from build123d import *

# Parameters (mm, degrees)
EXTRUDE_1_DEPTH     = 4
FILLET_1_R          = 0.5
FILLET_2_R          = 1
CUT_EXTRUDE_1_DEPTH = 0.5
SKETCH_3_W          = 3.444181234
SKETCH_3_H          = 7
SKETCH_3_W_2        = 2.596632025
CUT_EXTRUDE_2_DEPTH = 17


with BuildPart() as part:
    # 草图1 → 凸台-拉伸1 (new, symmetric)
    with BuildSketch(Plane.XY):
        Polygon((0, 0), (6.275985866, 3.1), (14.2, 2), (14.2, 20), (14.7, 20), (14.7, 1.425796077), (6.359548127, 2.583605352), (1.1290092, 0), (6.359548127, -2.583605352), (14.7, -1.425796077), (14.7, -20), (14.2, -20), (14.2, -2), (6.275985866, -3.1), align=None)
    extrude(amount=EXTRUDE_1_DEPTH, both=True)

    # 圆角1
    fillet_1_edges = [part.edges().sort_by_distance(p)[0] for p in [
        (14.2, 2, 0),
        (6.359548127, 2.583605352, 0),
        (1.1290092, 0, 0),
        (6.359548127, -2.583605352, 0),
        (14.2, -2, 0),
    ]]
    fillet(fillet_1_edges, radius=FILLET_1_R)

    # 圆角2
    fillet_2_edges = [part.edges().sort_by_distance(p)[0] for p in [
        (0, 0, 0),
        (6.275985866, 3.1, 0),
        (14.7, 1.425796077, 0),
        (14.7, -1.425796077, 0),
        (6.275985866, -3.1, 0),
    ]]
    fillet(fillet_2_edges, radius=FILLET_2_R)

    # 草图2 → 切除-拉伸1 (cut)
    with BuildSketch(Plane.ZY.offset(-14.2)):
        with BuildLine():
            Line((1.5, 16), (1.5, 12))
            ThreePointArc((1.5, 12), (0, 10.5), (-1.5, 12))
            Line((-1.5, 12), (-1.5, 16))
            ThreePointArc((-1.5, 16), (0, 17.5), (1.5, 16))
        make_face()
        with BuildLine():
            Line((1.5, -12), (1.5, -16))
            ThreePointArc((1.5, -16), (0, -17.5), (-1.5, -16))
            Line((-1.5, -16), (-1.5, -12))
            ThreePointArc((-1.5, -12), (0, -10.5), (1.5, -12))
        make_face()
    extrude(amount=-CUT_EXTRUDE_1_DEPTH, mode=Mode.SUBTRACT)

    # 草图3 → 切除-拉伸2 (cut, symmetric)
    with BuildSketch(Plane.ZY.offset(-14.2)):
        with Locations((4.722090617, 0)):
            Rectangle(SKETCH_3_W, SKETCH_3_H)
        with Locations((-4.298316013, 0)):
            Rectangle(SKETCH_3_W_2, SKETCH_3_H)
    extrude(amount=CUT_EXTRUDE_2_DEPTH, both=True, mode=Mode.SUBTRACT)


solid = part.part
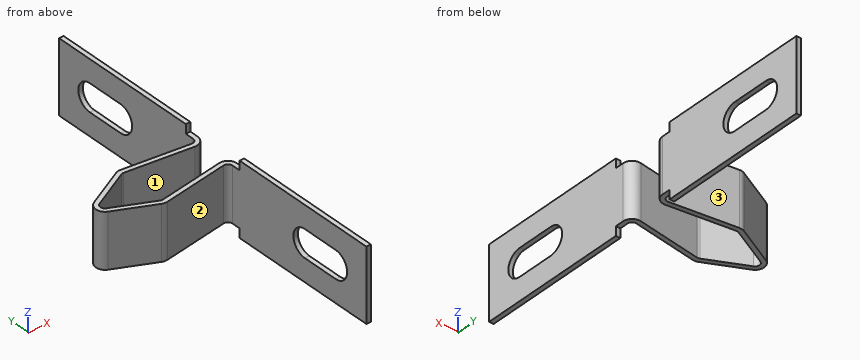
The listing builds one solid part. Answer for the finished solid, in the listing's coordinates (mm). Face numbers are marked on the shaded views. A direction names the side the tool comes from. Round coordinates to 2 decimals unless told otherwise and drop trailing zeros. Loops run counter-clockwise (first coordinate to the right, second up) from the corner with the lowest first, then second, coordinate; pieces in that order, holes last. Notation, with made-up numbers: M 56,-33.5 L 86,-33.5 A15 cw 86,-7.5 Z; hole C 18,-14 d8. An arc over 180 degrees is marked long. Return JSON: item names as keys, results as strings.
Q1. Find section B-B, the plane y = -17. Determine the outline of the cut face in (x, z), plus the area to 3 significant figures.
Results list:
{"outline": "M 14.2,-4 L 14.7,-4 L 14.7,-1.12 L 14.2,-1.12 Z; M 14.2,1.12 L 14.7,1.12 L 14.7,4 L 14.2,4 Z", "area": "2.88 mm2"}
Q2. Each of these flat-tipped pins is pushed along its axis until it touches: pin 1 Ø2 at (x, y) = (8.5, 2.5) entering from -Z; pin 2 Ø4 at (y, z) = (-12.5, -0.5) entering from -X; pin 3 Ø1.5 at (x, z) = (12, -1.5) entering from -Y. Where does it stop, or does it pass through?
Results list:
{"pin 1": "stops at z = -3", "pin 2": "stops at x = 14.2", "pin 3": "stops at y = -2.41"}
Q3. Find section D-D, the plane z = -2.25. Determine the outline of the cut face in (x, y).
Results list:
{"outline": "M 1.82,-0.9 L 6,-2.96 A1 ccw 6.58,-3.06 L 13.63,-2.08 A0.5 cw 14.2,-2.57 L 14.2,-20 L 14.7,-20 L 14.7,-2.57 A1 ccw 13.56,-1.58 L 6.51,-2.56 A0.5 cw 6.22,-2.52 L 2.04,-0.45 A0.5 cw 2.04,0.45 L 6.22,2.52 A0.5 cw 6.51,2.56 L 13.56,1.58 A1 ccw 14.7,2.57 L 14.7,20 L 14.2,20 L 14.2,2.57 A0.5 cw 13.63,2.08 L 6.58,3.06 A1 ccw 6,2.96 L 1.82,0.9 A1 ccw Z"}
Q4. Which of the six approach directions +Z, -Z, +X, -X, +Y, -Y give full straight-line access (tool end or side, diameter ignored) to the marked faces 1, 2 and 3?
Results list:
{"face 1": "+Z, -Z", "face 2": "+Z, -Z, -Y", "face 3": "+Z, -Z, +Y"}
Q5. Find section C-C, the plane x = 3. Determine the outline of the cut face in (y, z), plus the area to 3 significant figures.
Results list:
{"outline": "M -1.48,-3 L -0.92,-3 L -0.92,3 L -1.48,3 Z; M 0.92,-3 L 1.48,-3 L 1.48,3 L 0.92,3 Z", "area": "6.69 mm2"}
Q6. Find the intervals of material crossed by line 1 along Y through (x, z) = (2.25, 2.5); line 2 along Y through (x, z) = (6.75, 1.25); line 3 along X through (y, z) = (9, -3), in increasing order. Write a range as from..to.
Results list:
{"line 1": "y = -1.11..-0.55, 0.55..1.11", "line 2": "y = -3.03..-2.53, 2.53..3.03", "line 3": "x = 14.2..14.7"}
Q7. Find section A-A, the plane z = 0. State how many separate pieces and enclosed holes the cut face has, plus the area to 3 significant figures.
Results list:
{"separate pieces": "3", "enclosed holes": "0", "area": "24.8 mm2"}
